Geometry check sheet. Reference: the model listing, model coordinates, mm. A direction names the side the tool comes from. Coordinates: 2 decimals unless noted, no trailing zeros. Write each loop counter-clockwise with the first axis right and the second up, starting at its lowest first coordinate (ties: lowest second). Pieces come first, ordered by that corner, then holes. Notation, with made-up numbers: (9.5, 39) - (58.5, 39) arc R23 cw to (58.5, 77) - close; hole circle Ø1 at (40, -9). An arc over 180 degrees is marked (long way). Answer as a JSON object with one key per item and string values. Group by question number.
from build123d import *

# Parameters (mm, degrees)
SKETCH1_W           = 170
SKETCH1_H           = 170
BOSS_EXTRUDE2_DEPTH = 30
SKETCH2_R           = 5.1
CUT_EXTRUDE1_DEPTH  = 25
SKETCH3_R           = 5
SKETCH3_R_2         = 2.5
BOSS_EXTRUDE3_DEPTH = 10
FILLET1_R           = 10


with BuildPart() as part:
    # Sketch1 → Boss-Extrude2 (new body)
    with BuildSketch(Plane(origin=(0, 0, 0), x_dir=(1, 0, 0), z_dir=(0, 1, 0))):
        with Locations((85, 85)):
            Rectangle(SKETCH1_W, SKETCH1_H)
    extrude(amount=BOSS_EXTRUDE2_DEPTH)

    # Sketch2 → Cut-Extrude1 (cut)
    with BuildSketch(Plane(origin=(0, 30, 0), x_dir=(1, 0, 0), z_dir=(0, 1, 0))):
        with Locations((85, 12.5)):
            Circle(SKETCH2_R)
        with Locations((85, 157.5)):
            Circle(SKETCH2_R)
    extrude(amount=-CUT_EXTRUDE1_DEPTH, mode=Mode.SUBTRACT)

    # Sketch3 → Boss-Extrude3 (add)
    with BuildSketch(Plane(origin=(0, 30, 0), x_dir=(1, 0, 0), z_dir=(0, 1, 0))):
        with Locations((30, 30)):
            Circle(SKETCH3_R)
        with Locations((30, 30)):
            Circle(SKETCH3_R_2, mode=Mode.SUBTRACT)
        with Locations((140, 30)):
            Circle(SKETCH3_R)
        with Locations((140, 30)):
            Circle(SKETCH3_R_2, mode=Mode.SUBTRACT)
        with Locations((30, 140)):
            Circle(SKETCH3_R)
        with Locations((30, 140)):
            Circle(SKETCH3_R_2, mode=Mode.SUBTRACT)
        with Locations((140, 140)):
            Circle(SKETCH3_R)
        with Locations((140, 140)):
            Circle(SKETCH3_R_2, mode=Mode.SUBTRACT)
    extrude(amount=BOSS_EXTRUDE3_DEPTH)

    # Fillet1
    fillet1_edges = [part.edges().sort_by_distance(p)[0] for p in [
        (0, 15, -170),
        (170, 15, -170),
        (170, 15, 0),
        (0, 15, 0),
    ]]
    fillet(fillet1_edges, radius=FILLET1_R)


solid = part.part
(1) Gauge pin test, flat end, axial feed: pin 1 (3 mm diameter, centred on x = 73.5, z = -37.5, fed in from +Y). Record the tip position at first contact, or that the pin passes through.
(2) Section check A-A (x = 85). Record the cut outline in (y, z), and give its area (3 significant figures).
(3) Section check B-B (z = -30). Record the cut outline in (x, y), and give its area (3 significant figures).
(4) Draft check along Z on faces 3 (the face through (136, 35, -27)), 4 (the face through (166.99, 15.21, -167.15)), 5 (the face through (170, 15, -84)). Enter one of: +Z half, -Z half, draft (parallel to the pull), parting line (faces both ways), or undercut.
(5) Set-up check for faces 1 (the face through (2.85, 15.21, -3.01)), 2 (the face through (85, 5, -13)): record each of +Z, -Z, +X, -X, +Y, -Y from which the full face is reachable in a straight line by a thin tool's end or side.
(6) Material ranges on L1, parallel to X at y = 37, z = -30; L2, parallel to Z at x = 30, y = 37.5; L3, parallel to Z at x = 85, y = 18, recorded low to high. Write a range as [from, to].
(7) Section check C-C (x = 140). Record the cut outline in (y, z).
(8) Section check D-D (z = -157.5). Record the cut outline in (x, y), and give its area (4 significant figures).
Conclusion:
{
 "1": {"pin 1": "stops at y = 30"},
 "2": {"outline": "(0, -170) - (30, -170) - (30, -162.6) - (5, -162.6) - (5, -152.4) - (30, -152.4) - (30, -17.6) - (5, -17.6) - (5, -7.4) - (30, -7.4) - (30, 0) - (0, 0) - close", "area": "4,590 mm^2"},
 "3": {"outline": "(0, 0) - (170, 0) - (170, 30) - (145, 30) - (145, 40) - (142.5, 40) - (142.5, 30) - (137.5, 30) - (137.5, 40) - (135, 40) - (135, 30) - (35, 30) - (35, 40) - (32.5, 40) - (32.5, 30) - (27.5, 30) - (27.5, 40) - (25, 40) - (25, 30) - (0, 30) - close", "area": "5,200 mm^2"},
 "4": {"face 3": "undercut", "face 4": "-Z half", "face 5": "draft"},
 "5": {"face 1": "+Z, -X, +Y, -Y", "face 2": "+Y"},
 "6": {"L1": "x = [25, 27.5], [32.5, 35], [135, 137.5], [142.5, 145]", "L2": "z = [-145, -142.5], [-137.5, -135], [-35, -32.5], [-27.5, -25]", "L3": "z = [-170, -162.6], [-152.4, -17.6], [-7.4, 0]"},
 "7": {"outline": "(0, -170) - (30, -170) - (30, -145) - (40, -145) - (40, -142.5) - (30, -142.5) - (30, -137.5) - (40, -137.5) - (40, -135) - (30, -135) - (30, -35) - (40, -35) - (40, -32.5) - (30, -32.5) - (30, -27.5) - (40, -27.5) - (40, -25) - (30, -25) - (30, 0) - (0, 0) - close"},
 "8": {"outline": "(0, 0) - (170, 0) - (170, 30) - (90.1, 30) - (90.1, 5) - (79.9, 5) - (79.9, 30) - (0, 30) - close", "area": "4,845 mm^2"}
}
